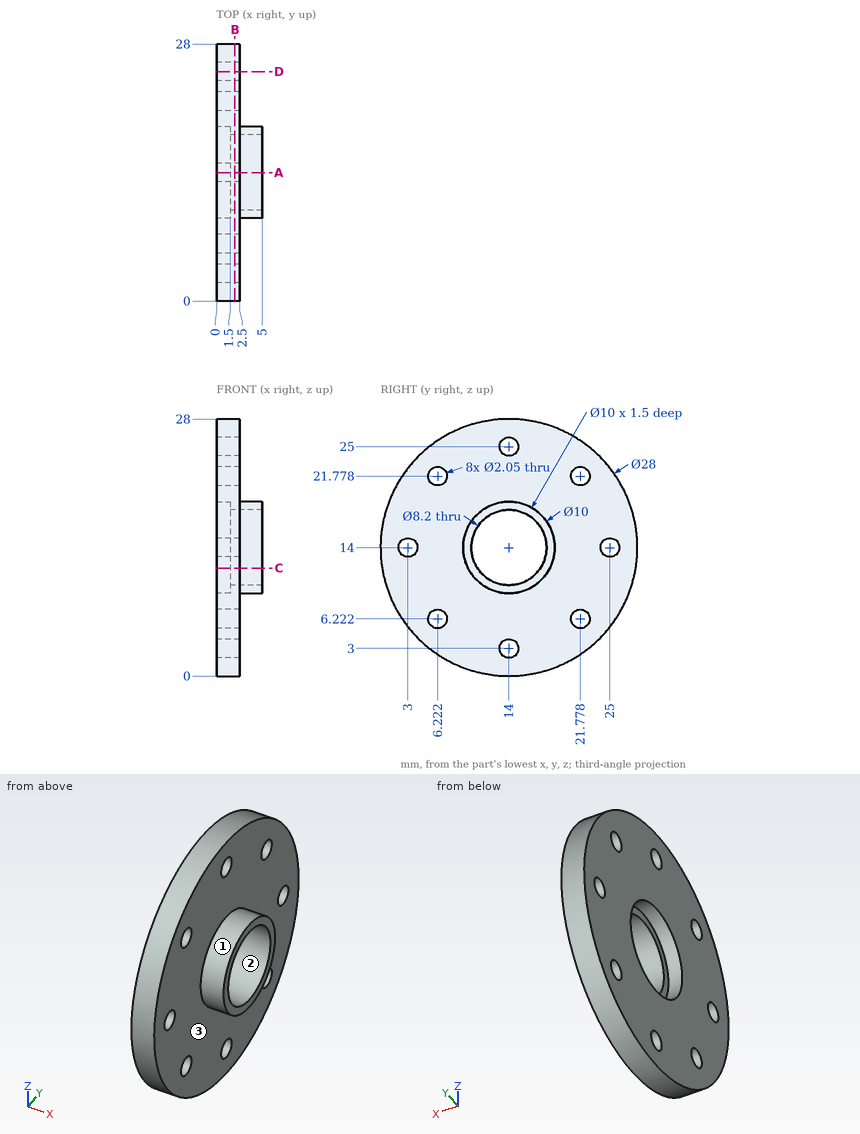
Geometry: see drawing. Coordinates: mm, zero at the bounding-box minimum. Round coordinates to 2 decimals unless told otherwise and drop trailing zeros. Loops run counter-clockwise (first coordinate to the right, second up) from the corner with the lowest first, then second, coordinate; pieces in that order, holes last.
(1) Contact query for flat-ended pins moving along their axis: pin 1 Ø3.5 at (y, z) = (14, 3) entering from +X; pin 2 Ø1 at (x, z) = (1.5, 18.5) entering from -Y; pin 3 Ø1.8 at (y, z) = (21.78, 21.78) entering from +X; pin 4 Ø1 at (x, y) = (3.5, 15.5) entering from -Z. Output: stop coordinate, or through.
From the geometry:
pin 1: stops at x = 2.5
pin 2: stops at y = 0.58
pin 3: passes through
pin 4: stops at z = 9.1
(2) Section query A-A (y = 14). Output: boundary loops of the cut face in (x, z) (3 decimals).
From the geometry:
outline: (0, 0) - (2.5, 0) - (2.5, 1.975) - (0, 1.975) - close; (0, 4.025) - (2.5, 4.025) - (2.5, 9) - (5, 9) - (5, 9.9) - (1.5, 9.9) - (1.5, 9) - (0, 9) - close; (0, 19) - (1.5, 19) - (1.5, 18.1) - (5, 18.1) - (5, 19) - (2.5, 19) - (2.5, 23.975) - (0, 23.975) - close; (0, 26.025) - (2.5, 26.025) - (2.5, 28) - (0, 28) - close
(3) Section query D-D (y = 25). Output: boundary loops of the cut face in (x, z) (1 decimal).
From the geometry:
outline: (0, 5.3) - (2.5, 5.3) - (2.5, 13) - (0, 13) - close; (0, 15) - (2.5, 15) - (2.5, 22.7) - (0, 22.7) - close
(4) Material intervals for probe 1 along Z at (x, y) = (1.15, 22); probe 2 along Z at (x, y) = (1, 5.75); probe 3 along Y at (x, z) = (0.3, 21.5) (1 decimal), sorted ascending.
From the geometry:
probe 1: z = 2.51 to 5.22, 7.22 to 20.78, 22.78 to 25.49
probe 2: z = 2.69 to 5.31, 7.13 to 20.87, 22.69 to 25.31
probe 3: y = 2.2 to 5.2, 7.2 to 20.8, 22.8 to 25.8
(5) Pull-direction query (Z, two-part tool) for the marked faces 1, 2 and 3; classes: +Z half, -Z half, draft (parallel to the pull), parting line (faces both ways), or undercut.
From the geometry:
face 1: parting line
face 2: undercut
face 3: draft
(6) Section query B-B (x = 2). Give the number of separate pieces and of enclosed holes in the cut face.
From the geometry:
separate pieces: 1
enclosed holes: 9
(7) Section query C-C (z = 11.75). Output: boundary loops of the cut face in (x, y) (1 decimal), and give its area (3 significant figures).
From the geometry:
outline: (0, 0.2) - (2.5, 0.2) - (2.5, 9.5) - (5, 9.5) - (5, 10.6) - (1.5, 10.6) - (1.5, 9.5) - (0, 9.5) - close; (0, 18.5) - (1.5, 18.5) - (1.5, 17.4) - (5, 17.4) - (5, 18.5) - (2.5, 18.5) - (2.5, 27.8) - (0, 27.8) - close
area: 54.0 mm2
